from build123d import *

# Parameters (mm, degrees)
ESQUISSE1_R                  = 20
BOSS_EXTRU_1_DEPTH           = 3.175
ESQUISSE2_R                  = 4.05
ESQUISSE2_R_2                = 0.9
ENL_V_MAT_EXTRU_1_DEPTH      = 29.461915343
ENL_V_MAT_EXTRU_2_DEPTH      = 29.461915343
ENL_V_MAT_EXTRU_2_DEPTH_BACK = 29.461915343
ESQUISSE3_R                  = 1.5


with BuildPart() as part:
    # Esquisse1 → Boss.-Extru.1 (new body)
    with BuildSketch(Plane.XY):
        Circle(ESQUISSE1_R)
    extrude(amount=BOSS_EXTRU_1_DEPTH)

    # Esquisse2 → Enlèv. mat.-Extru.1 (cut, through all)
    with BuildSketch(Plane.XY.offset(3.175)):
        Circle(ESQUISSE2_R)
        with Locations((0, 8)):
            Circle(ESQUISSE2_R_2)
        with Locations((8, 0)):
            Circle(ESQUISSE2_R_2)
        with Locations((0, -8)):
            Circle(ESQUISSE2_R_2)
        with Locations((-8, 0)):
            Circle(ESQUISSE2_R_2)
    extrude(amount=-ENL_V_MAT_EXTRU_1_DEPTH, mode=Mode.SUBTRACT)

    # Esquisse3 → Enlèv. mat.-Extru.2 (cut, two sides: drawn at the far end of the back side and taken through both)
    with BuildSketch(Plane.XY.offset(3.175).offset(-ENL_V_MAT_EXTRU_2_DEPTH_BACK)):
        with Locations((10.606601718, 10.606601718)):
            Circle(ESQUISSE3_R)
        with Locations((10.606601718, -10.606601718)):
            Circle(ESQUISSE3_R)
        with Locations((-10.606601718, -10.606601718)):
            Circle(ESQUISSE3_R)
        with Locations((-10.606601718, 10.606601718)):
            Circle(ESQUISSE3_R)
    extrude(amount=ENL_V_MAT_EXTRU_2_DEPTH + ENL_V_MAT_EXTRU_2_DEPTH_BACK, mode=Mode.SUBTRACT)


solid = part.part
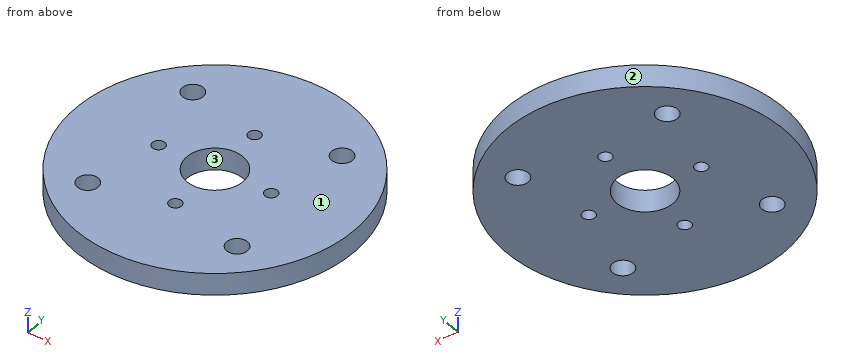
Source: CAD feature listing. Evaluate the final solid. Frame: model axes, mm. Face numbers are marked on the shaded views. Round coordinates to 2 decimals unless told otherwise and drop trailing zeros. Write each loop counter-clockwise with the first axis right and the second up, starting at its lowest first coordinate (ties: lowest second). Pieces come first, ordered by that corner, then holes. Notation, with made-up numbers: (14, 1) - (49, 1) arc R12 ccw to (49, 19) - close; hole circle Ø4 at (-38, 47.5). An arc over 180 degrees is marked (long way). Use CSV: the item, a comma, the result in double quotes. Start each with the question number.
(1) Material intervals for probe 1 along Y at (x, z) = (0, 1.95); probe 2 along X at (y, z) = (-10, 1.7); probe 3 along X at (y, z) = (-0.5, 1.75), sorted ascending. Write a range as [from, to].
(2) Cut plane D-D, the plane z = 0.8. Give the number of separate pieces and of enclosed holes in the cut face, and give its area (3 significant figures).
(3) Cut plane A-A, the plane x = -8. Return loops of the section in (y, z) (3 decimals), and give its area (3 significant figures).
(4) Cut plane C-C, the plane y = 10. Return loops of the section in (x, z) (1 decimal).
(5) Mould query, pull axis X, two halves, no side actions, for the marked faces 1, 2 and 3. Classes: pulls with the +X half, pulls with the -X half, needs draft (parallel to the pull), parting line crosses it, or undercut.
(6) First-contact query: pin 1 Ø1.5 at (y, z) = (-14, 2) entering from -X. Flat tip, straight axial feed; report the tip coordinate or a pass-through.
Geometry says:
1,probe 1,"[-20, -8.9], [-7.1, -4.05], [4.05, 7.1], [8.9, 20]"
1,probe 2,"[-17.32, -11.98], [-9.23, 9.23], [11.98, 17.32]"
1,probe 3,"[-19.99, -8.75], [-7.25, -4.02], [4.02, 7.25], [8.75, 19.99]"
2,separate pieces,"1"
2,enclosed holes,"9"
2,area,"1,170 mm²"
3,outline,"(-18.33, 0) - (-0.9, 0) - (-0.9, 3.175) - (-18.33, 3.175) - close; (0.9, 0) - (18.33, 0) - (18.33, 3.175) - (0.9, 3.175) - close"
3,area,"111 mm²"
4,outline,"(-17.3, 0) - (-12, 0) - (-12, 3.2) - (-17.3, 3.2) - close; (-9.2, 0) - (9.2, 0) - (9.2, 3.2) - (-9.2, 3.2) - close; (12, 0) - (17.3, 0) - (17.3, 3.2) - (12, 3.2) - close"
5,face 1,"needs draft"
5,face 2,"parting line crosses it"
5,face 3,"undercut"
6,pin 1,"x = -14.98"
